Autodesk Inventor part; units mm, degrees
ref_plane "YZ Plane" through (0, 0, 0) normal (1, 0, 0) x (0, 1, 0)
ref_plane "XZ Plane" through (0, 0, 0) normal (0, 1, 0) x (-1, 0, 0)
ref_plane "XY Plane" through (0, 0, 0) normal (0, 0, 1) x (1, 0, 0)
sketch "Sketch1" plane through (0, 0, 0) normal (0, 0, 1) x (1, 0, 0)
  line L0 (50, -50) -> (-50, -50)
  line L1 (50, 50) -> (50, -50)
  line L2 (50, 50) -> (-10, 50)
  line L3 (-10, 50) -> (-50, -50)
  line L4 (-10, 50) -> (20, 50)
  line L5 (20, 50) -> (50, 50)
  line L6 (-1, 45) -> (11, 45)
  line L7 (11, 45) -> (11, 55)
  line L8 (11, 55) -> (-1, 55)
  line L9 (-1, 55) -> (-1, 45)
  line L10 (-1, 45) -> (11, 55) construction
  line L11 (11, 45) -> (-1, 55) construction
  line L12 (50, 50) -> (37.9, 50)
  line L13 (31.9, 45) -> (43.9, 45)
  line L14 (43.9, 45) -> (43.9, 55)
  line L15 (43.9, 55) -> (31.9, 55)
  line L16 (31.9, 55) -> (31.9, 45)
  line L17 (31.9, 45) -> (43.9, 55) construction
  line L18 (43.9, 45) -> (31.9, 55) construction
  line L19 (-3, 50) -> (-3, 43)
  line L20 (-3, 43) -> (13, 43)
  line L21 (13, 43) -> (13, 50)
  line L22 (29.9, 50) -> (29.9, 43)
  line L23 (29.9, 43) -> (45.9, 43)
  line L24 (45.9, 43) -> (45.9, 50)
  point P0 (0, 0)
  point P1 (5, 50)
  point P2 (-1, 50)
  point P3 (45.9, 46.5)
  point P4 (31.9, 50)
  point P5 (43.9, 50)
  point P6 (-1, 50)
  point P7 (11, 50)
  dimension "d18" = 60
  dimension "d19" = 111.801
  dimension "d20" = 100
  dimension "d21" = 100
  dimension "d22" = 50
  dimension "d23" = 50
  dimension "d24" = 30
  dimension "d25" = 12
  dimension "d26" = 10
  dimension "d31" = 12.1
  dimension "d32" = 12
  dimension "d33" = 10
  dimension "d36" = 2
  dimension "d37" = 2
  dimension "d38" = 16
  dimension "d39" = 2
  dimension "d40" = 2
  dimension "d41" = 2
extrude "Extrusion1" add sketch "Sketch1" along normal blind 3 contours L0 L3 L2 L19 L20 L21 L22 L23 L24 L1 | L24 L23 L22 L2 L16 L13 L14 | L2 L9 L6 L7 L21 L20 L19 | L14 L13 L16 L2 | L2 L7 L6 L9
extrude "Extrusion2" cut sketch "Sketch1" along normal blind 10 contours L9 L8 L7 L2 | L2 L7 L6 L9
extrude "Extrusion3" cut sketch "Sketch1" along normal blind 10 contours L14 L13 L16 L2 | L2 L16 L15 L14
extrude "Extrusion4" add sketch "Sketch1" against normal blind 20 contours L24 L23 L22 L2 L16 L13 L14 | L2 L9 L6 L7 L21 L20 L19
sketch "Sketch2" plane through (0, 0, 0) normal (0, 0, 1) x (1, 0, 0)
  line L0 (-52.1328, -49.9469) -> (-12.1328, 50.0531)
  line L1 (-10, 50) -> (-50, -50)
  line L2 (-1, 50) -> (-10, 50)
  line L3 (-12.1328, 50.0531) -> (-21.8999, 50.0531)
  line L4 (-21.8999, 50.0531) -> (-21.8999, 45)
  line L5 (-21.8999, 45) -> (-33.8999, 45)
  line L6 (-33.8999, 45) -> (-33.8999, 50.0531)
  line L7 (-33.8999, 50.0531) -> (-41.8999, 50.0531)
  line L8 (-52.1328, -49.9469) -> (-67.1328, -49.9469)
  line L9 (-67.1328, -49.9469) -> (-67.1328, -9.9469)
  line L10 (-67.1328, -9.9469) -> (-41.8999, 50.0531)
  line L11 (-67.1328, -4.7877) -> (-44.0696, 50.0531)
  line L12 (-67.1328, -4.7877) -> (-67.1328, 50.0531)
  line L13 (-67.1328, 50.0531) -> (-64.1328, 50.0531)
  line L14 (-64.1328, 50.0531) -> (-64.1328, 45.0531)
  line L15 (-64.1328, 45.0531) -> (-52.1328, 45.0531)
  line L16 (-52.1328, 45.0531) -> (-52.1328, 50.0531)
  line L17 (-52.1328, 50.0531) -> (-44.0696, 50.0531)
  line L18 (-50, -50) -> (50, -50)
  point P0 (0, 0)
  dimension "d44" = 20.9
  dimension "d46" = 12
  dimension "d47" = 8
  dimension "d48" = 15
  dimension "d49" = 40
  dimension "d50" = 2
  dimension "d51" = 2
  dimension "d52" = 3
  dimension "d53" = 5
  dimension "d54" = 12
  dimension "d55" = 54.8409
  dimension "d56" = 8.0632
  dimension "d57" = 67.191
  dimension "d58" = 9.7671
  dimension "d59" = 60
  dimension "d60" = 117.1328
  dimension "d61" = 5
properties part number "BasePart"
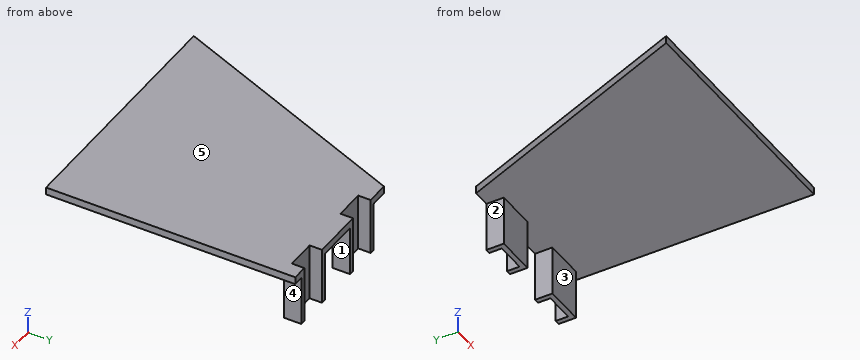
The model under review builds one solid part; all positions refer to its coordinate system, in mm. Face numbers are marked on the shaded views. A direction names the side the tool comes from. Round coordinates to 2 decimals unless told otherwise and drop trailing zeros. Loops run counter-clockwise (first coordinate to the right, second up) from the corner with the lowest first, then second, coordinate; pieces in that order, holes last. Notation, with made-up numbers: (64, 37.5) -> (121, 37.5) arc R17 cw to (121, 62.5) -> close; hole circle Ø9 at (-35, 9.25). An arc over 180 degrees is marked (long way). One line per question, with ' | ' between items. Start each with the question number.
Item 1: Add section C-C, the plane y = 25. Write out the cut boundary in (x, z), then the cut area to 3 significant figures.
Item 2: Machinability: for the marked faces 1, 2, 3, 4 and 5, which of the approach directions +Z, -Z, +X, -X, +Y, -Y give a long, thin tool a straight path to every point of the face, cutting with its end or side? Answer none if there is none.
Item 3: Add section B-B, the plane x = 39. Write out the cut boundary in (y, z), then the cut area to 3 significant figures.
Item 4: For pin 1 (7.5 mm diameter, centred on y = 45, z = -12.5, fed in from +X); pin 2 (2.5 mm diameter, centred on y = 47.5, z = -11.5, fed in from -X); pin 3 (6 mm diameter, centred on x = 38.5, z = -3, fed in from +Y), all flat-tipped, find the tip position at first contact; note any pin that passes through.
Item 5: Add section A-A, the plane z = -2.25. Write out the cut boundary in (x, y).
Item 6: Wall thickness on line 1 along Z through (x, y) = (-2, -39.5); line 2 along Y through (x, z) = (32, -13.5); line 3 along Y through (x, z) = (4, 0.75): over which ranges is each line inside the solid? List them lowest first. Write a range as [from, to].
Item 7: Add section D-D, the plane x = -14. Write out the cut boundary in (y, z), then the cut area to 3 significant figures.
Return value:
1) outline: (-20, 0) -> (50, 0) -> (50, 3) -> (-20, 3) -> close | area: 210 mm2
2) face 1: -Z, +Y, -Y | face 2: -Z, -X, +Y, -Y | face 3: -Z, +X, -X, -Y | face 4: -Z, +X, +Y, -Y | face 5: +Z, +X, -X, +Y, -Y
3) outline: (-50, 0) -> (43, 0) -> (43, -20) -> (45, -20) -> (45, 3) -> (-50, 3) -> close | area: 325 mm2
4) pin 1: stops at x = 45.9 | pin 2: stops at x = -3 | pin 3: stops at y = 45
5) outline: (-3, 43) -> (13, 43) -> (13, 50) -> (11, 50) -> (11, 45) -> (-1, 45) -> (-1, 50) -> (-3, 50) -> close; (29.9, 43) -> (45.9, 43) -> (45.9, 50) -> (43.9, 50) -> (43.9, 45) -> (31.9, 45) -> (31.9, 50) -> (29.9, 50) -> close
6) line 1: z = [0, 3] | line 2: y = [43, 45] | line 3: y = [-50, 45]
7) outline: (-50, 0) -> (40, 0) -> (40, 3) -> (-50, 3) -> close | area: 270 mm2
